For this review, take the finished solid that the model builds, in its own axes (mm). A direction names the side the tool comes from. Coordinates: 2 decimals unless noted, no trailing zeros. Loops run counter-clockwise (first coordinate to the right, second up) from the corner with the lowest first, then second, coordinate; pieces in that order, holes last. Notation, with made-up numbers: M 66,13.25 L 95,13.25 A11 cw 95,33.25 Z; hole C 7,-32.75 d11. An arc over 180 degrees is marked long. Write item = value, one per line.
from build123d import *

# Parameters (mm, degrees)
SKETCH_1_R      = 1.1
EXTRUDE_1_DEPTH = 1.6


with BuildPart() as part:
    # 草图1 → 凸台-拉伸1 (new body)
    with BuildSketch(Plane(origin=(0, 0, 0), x_dir=(1, 0, 0), z_dir=(0, 1, 0))):
        with BuildLine():
            ThreePointArc((0, 1.25), (0.366116524, 0.366116524), (1.25, 0))
            Line((1.25, 0), (78.95, 0))
            ThreePointArc((78.95, 0), (79.833883476, 0.366116524), (80.2, 1.25))
            Line((80.2, 1.25), (80.2, 31.65))
            ThreePointArc((80.2, 31.65), (79.833883476, 32.533883476), (78.95, 32.9))
            Line((78.95, 32.9), (59.6, 32.9))
            ThreePointArc((59.6, 32.9), (59.175735931, 32.724264069), (59, 32.3))
            Line((59, 32.3), (59, 31.5))
            ThreePointArc((59, 31.5), (58.824264069, 31.075735931), (58.4, 30.9))
            Line((58.4, 30.9), (47.6, 30.9))
            ThreePointArc((47.6, 30.9), (47.175735931, 31.075735931), (47, 31.5))
            Line((47, 31.5), (47, 32.3))
            ThreePointArc((47, 32.3), (46.824264069, 32.724264069), (46.4, 32.9))
            Line((46.4, 32.9), (1.25, 32.9))
            ThreePointArc((1.25, 32.9), (0.366116524, 32.533883476), (0, 31.65))
            Line((0, 31.65), (0, 30.5))
            ThreePointArc((0, 30.5), (-0.366116524, 29.616116524), (-1.25, 29.25))
            Line((-1.25, 29.25), (-8.95, 29.25))
            ThreePointArc((-8.95, 29.25), (-9.833883476, 28.883883476), (-10.2, 28))
            Line((-10.2, 28), (-10.2, 4.9))
            ThreePointArc((-10.2, 4.9), (-9.833883476, 4.016116524), (-8.95, 3.65))
            Line((-8.95, 3.65), (-1.25, 3.65))
            ThreePointArc((-1.25, 3.65), (-0.366116524, 3.283883476), (0, 2.4))
            Line((0, 2.4), (0, 1.25))
        make_face()
        with Locations((2.35, 3)):
            Circle(SKETCH_1_R, mode=Mode.SUBTRACT)
        with Locations((77.85, 3)):
            Circle(SKETCH_1_R, mode=Mode.SUBTRACT)
        with Locations((2.35, 29.9)):
            Circle(SKETCH_1_R, mode=Mode.SUBTRACT)
        with Locations((77.85, 29.9)):
            Circle(SKETCH_1_R, mode=Mode.SUBTRACT)
    extrude(amount=EXTRUDE_1_DEPTH)


solid = part.part
Q1. Add section C-C (x = 55). Write out the cut boundary in (y, z), and give its area (3 significant figures).
Solved:
outline = M 0,-30.9 L 1.6,-30.9 L 1.6,0 L 0,0 Z
area = 49.4 mm²
Q2. For line 1 along Z through (x, y) = (77.85, 0.8); line 2 along X through (y, z) = (0.5, -30); line 3 along X through (y, z) = (1, -29.9), list the stretches that pass through material, from the lowest coordinate up.
Solved:
line_1 = -32.9 to -31, -28.8 to -4.1, -1.9 to 0
line_2 = -0.1 to 1.25, 3.45 to 76.75, 78.95 to 80.2
line_3 = -0.15 to 1.25, 3.45 to 76.75, 78.95 to 80.2
Q3. Add section A-A (x = 77.85). Write out the cut boundary in (y, z).
Solved:
outline = M 0,-32.9 L 1.6,-32.9 L 1.6,-31 L 0,-31 Z; M 0,-28.8 L 1.6,-28.8 L 1.6,-4.1 L 0,-4.1 Z; M 0,-1.9 L 1.6,-1.9 L 1.6,0 L 0,0 Z
Q4. Add section B-B (y = 0.65). Write out the cut boundary in (x, z), and give its area (3 significant figures).
Solved:
outline = M -10.2,-28 A1.25 ccw -8.95,-29.25 L -1.25,-29.25 A1.25 cw 0,-30.5 L 0,-31.65 A1.25 ccw 1.25,-32.9 L 46.4,-32.9 A0.6 ccw 47,-32.3 L 47,-31.5 A0.6 cw 47.6,-30.9 L 58.4,-30.9 A0.6 cw 59,-31.5 L 59,-32.3 A0.6 ccw 59.6,-32.9 L 78.95,-32.9 A1.25 ccw 80.2,-31.65 L 80.2,-1.25 A1.25 ccw 78.95,0 L 1.25,0 A1.25 ccw 0,-1.25 L 0,-2.4 A1.25 cw -1.25,-3.65 L -8.95,-3.65 A1.25 ccw -10.2,-4.9 Z; hole C 2.35,-29.9 d2.2; hole C 2.35,-3 d2.2; hole C 77.85,-29.9 d2.2; hole C 77.85,-3 d2.2
area = 2,860 mm²
Q5. For pin 1 Ø3 at (x, z) = (2.35, -3) entering from -Y; pin 2 Ø0.5 at (x, y) = (-5.5, 1) entering from -Z; pin 3 Ø0.6 at (y, z) = (1, -2) entering from -X; pin 4 Ø0.8 at (x, y) = (53, 0.5) entering from -Z, all flat-tipped, find the tip position at first contact; note any pin that passes through.
Solved:
pin_1 = 0
pin_2 = -29.25
pin_3 = 0
pin_4 = -30.9
Q6. Machinability: for faces 4 (the face through (-5, 1, -3.65)), 5 (the face through (34, 1.6, -17)), which of the approach directions +Z, -Z, +X, -X, +Y, -Y give a long, thin tool a straight path to every point of the face, cutting with its end or side? Answer none if there is none.
Solved:
face_4 = +Z, -X, +Y, -Y
face_5 = +Z, -Z, +X, -X, +Y
Q7. Draft analysis for pull direction X (two halves, no side actions). For faces 1 (the face through (80.2, 1, -16)), 2 (the face through (-5, 1, -29.25)), 3 (the face through (53, 1, -30.9)), state which applies: +X half, -X half, draft (parallel to the pull), parting line (faces both ways), or undercut.
Solved:
face_1 = +X half
face_2 = draft
face_3 = undercut
